Geometry: final body of the model. Coordinates: model frame, mm. Coordinates: 2 decimals unless noted, no trailing zeros. Loops run counter-clockwise (first coordinate to the right, second up) from the corner with the lowest first, then second, coordinate; pieces in that order, holes last. Notation, with made-up numbers: (89, -37) -> (135, -37) arc R17 cw to (135, -32) -> close; hole circle Ø1 at (71, -19.75). An arc over 180 degrees is marked (long way). One line per item, written item: value. Start each with the question number.
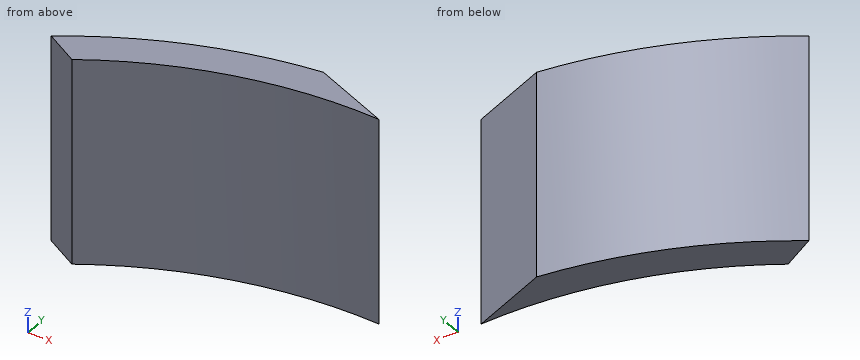
from build123d import *

# Parameters (mm, degrees)
BOSS_EXTRUDE1_DEPTH = 210
CUT_EXTRUDE1_REACH  = 379.535
CUT_EXTRUDE2_REACH  = 377.003


with BuildPart() as part:
    # Sketch1 → Boss-Extrude1 (new body)
    with BuildSketch(Plane.XY):
        with BuildLine():
            Line((0, 0), (0, -33.45))
            ThreePointArc((0, -33.45), (-142.866754092, -51.269235769), (-272.793704391, -113.296827807))
            Line((-272.793704391, -113.296827807), (-292.568960472, -86.318285465))
            ThreePointArc((-292.568960472, -86.318285465), (-153.270771234, -19.479665275), (0, 0))
        make_face()
    extrude(amount=BOSS_EXTRUDE1_DEPTH)

    # Sketch3 → Cut-Extrude1 (cut, up to next)
    with BuildSketch(Plane(origin=(0, 0, 0), x_dir=(-1, 0, 0), z_dir=(0, 0, -1)), mode=Mode.PRIVATE) as cut_extrude1_sk1:
        Polygon((292.568960472, -86.318285465), (255.457097019, -106.893394239), (272.793704391, -113.296827807), align=None)
    cut_extrude1_tool1 = extrude(cut_extrude1_sk1.sketch, amount=-CUT_EXTRUDE1_REACH, mode=Mode.PRIVATE) & part.part
    add(cut_extrude1_tool1.solids().sort_by_distance((-273.606587, -102.169503, 0))[0], mode=Mode.SUBTRACT)

    # Sketch4 → Cut-Extrude2 (cut, up to next)
    with BuildSketch(Plane(origin=(0, 0, 0), x_dir=(-1, 0, 0), z_dir=(0, 0, -1)), mode=Mode.PRIVATE) as cut_extrude2_sk1:
        Polygon((0, -33.45), (84.004446004, 0), (0, 0), align=None)
    cut_extrude2_tool1 = extrude(cut_extrude2_sk1.sketch, amount=-CUT_EXTRUDE2_REACH, mode=Mode.PRIVATE) & part.part
    add(cut_extrude2_tool1.solids().sort_by_distance((-28.001482, -11.15, 0))[0], mode=Mode.SUBTRACT)


with BuildPart() as cut_extrude2_kept_piece:
    # of the separate pieces the step leaves, the one the design keeps (cut_extrude2_pieces_kept)
    add(part.part.solids().sort_by_distance((-292.568960472, -86.318285465, 0))[0])


solid = cut_extrude2_kept_piece.part
1. Line query: L1, parallel to Y at x = -184.5, z = 14; L2, parallel to Y at x = -84.5, z = 20; L3, parallel to X at y = -98, z = 147. Output: solid intervals per line, ascending. Write a range as [from, to].
2. Section A-A on z = 161.5. Return the cut outline in (x, y), plus the area to 3 significant figures.
3. Section B-B on x = -49. Return the cut outline in (y, z), plus the area to 3 significant figures.
4. Pin query (flat end, axial travel): pin 1 Ø8 at (x, y) = (-203.5, -29.5) entering from +Z; pin 2 Ø1.5 at (x, z) = (-205.5, 87) entering from -Y; pin 3 Ø1.5 at (y, z) = (-57.5, 71) entering from -X; pin 4 Ø3 at (y, z) = (-80.5, 32) entering from -X. Return the tip coordinate at first contact, or that it passes through.
Checks:
1. L1: [-65.7, -29.86]
1. L2: [-38.32, -4.53]
1. L3: [-271.5, -249.18]
2. outline: (-292.57, -86.32) -> (-259.69, -104.55) arc R450 cw to (0, -33.45) -> (-75.59, -3.35) arc R483.45 ccw to start
2. area: 8,420 mm²
3. outline: (-34.33, 0) -> (-13.94, 0) -> (-13.94, 210) -> (-34.33, 210) -> close
3. area: 4,280 mm²
4. pin 1: through
4. pin 2: y = -75.13
4. pin 3: x = -247.05
4. pin 4: x = -286.26
